Build history of the part. All positions in model axes, mm. Face numbers are marked on the shaded views. A direction names the side the tool comes from. Round coordinates to 2 decimals unless told otherwise and drop trailing zeros. Order: outer loops, then holes, each group sorted by start corner. A loop starts at its lowest first (then second) coordinate and runs counter-clockwise, first axis right, second up. Notation, with made-up numbers: M 84,53 L 104,53 A13 cw 104,62 Z; hole C -27.75,-25 d8. An arc over 180 degrees is marked long. Use CSV: the item, a comma, the result in double quotes.
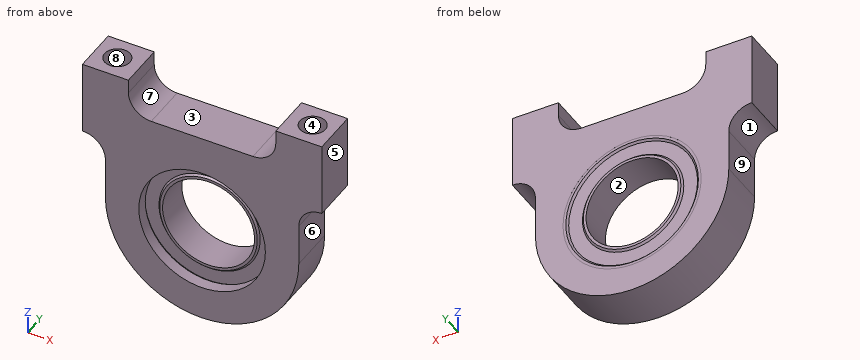
from build123d import *

# Parameters (mm, degrees)
SKETCH1_R                       = 8.73125
BOSS_EXTRUDE1_DEPTH             = 6.35
SKETCH2_R                       = 9.525
CUT_EXTRUDE1_DEPTH              = 4.7625
SKETCH3_R                       = 9.525
SKETCH3_R_2                     = 8.89
BOSS_EXTRUDE2_DEPTH             = 4.75996
CHAMFER1_SIZE                   = 0.254
SKETCH5_R                       = 6.985
SKETCH5_R_2                     = 6.35
BOSS_EXTRUDE3_DEPTH             = 4.75996
CHAMFER2_SIZE                   = 0.254
SKETCH6_R                       = 8.89
SKETCH6_R_2                     = 6.985
BOSS_EXTRUDE4_DEPTH             = 4.25196
F_6_32_TAPPED_HOLE1_D           = 2.7051
F_6_32_TAPPED_HOLE1_DEPTH       = 9.398
F_6_32_TAPPED_HOLE1_CBORE_D     = 3.5052
F_6_32_TAPPED_HOLE1_CBORE_DEPTH = 7.0104
F_6_32_TAPPED_HOLE1_TIP         = 0.81269403


with BuildPart() as part:
    # Sketch1 → Boss-Extrude1 (new body)
    with BuildSketch(Plane(origin=(0, 0, 0), x_dir=(1, 0, 0), z_dir=(0, 1, 0))):
        with BuildLine():
            Line((-13.335, 0), (-13.335, -5.7404))
            ThreePointArc((-13.335, -5.7404), (-14.257496482, -7.967503518), (-16.4846, -8.89))
            Line((-16.4846, -8.89), (-16.51, -8.89))
            Line((-16.51, -8.89), (-16.51, -19.05))
            Line((-16.51, -19.05), (-10.16, -19.05))
            Line((-10.16, -19.05), (-10.16, -17.1196))
            ThreePointArc((-10.16, -17.1196), (-9.237503518, -14.892496482), (-7.0104, -13.97))
            Line((-7.0104, -13.97), (7.0104, -13.97))
            ThreePointArc((7.0104, -13.97), (9.237503518, -14.892496482), (10.16, -17.1196))
            Line((10.16, -17.1196), (10.16, -19.05))
            Line((10.16, -19.05), (16.51, -19.05))
            Line((16.51, -19.05), (16.51, -8.89))
            Line((16.51, -8.89), (16.4846, -8.89))
            ThreePointArc((16.4846, -8.89), (14.257496482, -7.967503518), (13.335, -5.7404))
            Line((13.335, -5.7404), (13.335, 0))
            ThreePointArc((13.335, 0), (0, 13.335), (-13.335, 0))
        make_face()
        Circle(SKETCH1_R, mode=Mode.SUBTRACT)
    extrude(amount=BOSS_EXTRUDE1_DEPTH)

    # Sketch2 → Cut-Extrude1 (cut)
    with BuildSketch(Plane(origin=(0, 6.35, 0), x_dir=(1, 0, 0), z_dir=(0, 1, 0))):
        Circle(SKETCH2_R)
    extrude(amount=-CUT_EXTRUDE1_DEPTH, mode=Mode.SUBTRACT)

    # Sketch3 → Boss-Extrude2 (add)
    with BuildSketch(Plane(origin=(0, 1.5875, 0), x_dir=(-1, 0, 0), z_dir=(0, 1, 0))):
        Circle(SKETCH3_R)
        Circle(SKETCH3_R_2, mode=Mode.SUBTRACT)
    extrude(amount=BOSS_EXTRUDE2_DEPTH)

    # Chamfer1
    chamfer1_edges = [part.edges().sort_by_distance(p)[0] for p in [
        (8.89, 6.34746, 0),
    ]]
    chamfer(chamfer1_edges, length=CHAMFER1_SIZE)



with BuildPart() as body_2:
    # Sketch5 → Boss-Extrude3 (new body)
    with BuildSketch(Plane(origin=(0, 1.5875, 0), x_dir=(-1, 0, 0), z_dir=(0, 1, 0))):
        Circle(SKETCH5_R)
        Circle(SKETCH5_R_2, mode=Mode.SUBTRACT)
    extrude(amount=BOSS_EXTRUDE3_DEPTH)

    # Chamfer2
    chamfer2_edges = [body_2.edges().sort_by_distance(p)[0] for p in [
        (6.985, 1.5875, 0),
        (6.985, 6.34746, 0),
    ]]
    chamfer(chamfer2_edges, length=CHAMFER2_SIZE)


with BuildPart() as part_1:
    add(part.part)

    add(body_2.part)  # Boss-Extrude4 merges body 2
    # Sketch6 → Boss-Extrude4 (add)
    with BuildSketch(Plane(origin=(0, 6.09346, 0), x_dir=(-1, 0, 0), z_dir=(0, 1, 0))):
        Circle(SKETCH6_R)
        Circle(SKETCH6_R_2, mode=Mode.SUBTRACT)
    extrude(amount=-BOSS_EXTRUDE4_DEPTH)

    # #6-32 Tapped Hole1
    with Locations(Plane.XY.offset(19.05)):
        with Locations((-13.470384182, 3.175), (13.470384182, 3.175)):
            CounterBoreHole(F_6_32_TAPPED_HOLE1_D / 2, F_6_32_TAPPED_HOLE1_CBORE_D / 2, F_6_32_TAPPED_HOLE1_CBORE_DEPTH, depth=F_6_32_TAPPED_HOLE1_DEPTH)
            with Locations((0, 0, -(F_6_32_TAPPED_HOLE1_DEPTH + F_6_32_TAPPED_HOLE1_TIP / 2))):  # 118° drill point
                Cone(0, F_6_32_TAPPED_HOLE1_D / 2, F_6_32_TAPPED_HOLE1_TIP, mode=Mode.SUBTRACT)


solid = part_1.part
(1) Tool access for the marked faces 5, 6, 7, 8 and 9: list every direction of +Z, -Z, +X, -X, +Y, -Y with a clear straight run to the whole face (end or side of a thin tool).
Answer block:
face 5,"+Z, -Z, +X, +Y, -Y"
face 6,"-Z, +X, +Y, -Y"
face 7,"+Z, +Y, -Y"
face 8,"+Z"
face 9,"-Z, -X, +Y, -Y"
(2) Two-plate mould, pull along Z, no slides. Class the marked faces 1, 2, 3 and 4: released by +Z, released by -Z, zero draft, split by the parting line, or undercut.
Answer block:
face 1,"released by -Z"
face 2,"undercut"
face 3,"released by +Z"
face 4,"zero draft"
(3) Cut at C-C, the plane z = 14.5. Give the cut face in (x, y) (3 decimals), and give its area (3 significant figures).
Answer block:
outline,"M -16.51,0 L -8.759,0 L -8.759,6.35 L -16.51,6.35 Z; M 8.759,0 L 16.51,0 L 16.51,6.35 L 8.759,6.35 Z; hole C -13.47,3.175 d3.505; hole C 13.47,3.175 d3.505"
area,"79.1 mm²"
(4) Cut at D-D, the plane y = 5.5. Give the cut face in (x, z) (3 decimals), and give its area (3 significant figures).
Answer block:
outline,"M -16.51,8.89 L -16.485,8.89 A3.15 cw -13.335,5.74 L -13.335,0 A13.335 ccw 13.335,0 L 13.335,5.74 A3.15 cw 16.485,8.89 L 16.51,8.89 L 16.51,19.05 L 10.16,19.05 L 10.16,17.12 A3.15 cw 7.01,13.97 L -7.01,13.97 A3.15 cw -10.16,17.12 L -10.16,19.05 L -16.51,19.05 Z; hole C 0,0 d12.7"
area,"631 mm²"
(5) Drop flat-ended pins along their axis: pin 1 (7.5 mm diameter, centred on x = 0, z = 0, fed in from +Y); pin 2 (15 mm diameter, centred on x = 0.5, z = 1, fed in from -Y); pin 3 (1.8 mm diameter, centred on x = 13, y = 3, fed in from +Z); pin 4 (2 mm diameter, centred on y = 0.5, z = 6, fed in from +X). Give the stop position or say it passes through.
Answer block:
pin 1,"passes through"
pin 2,"stops at y = 1.59"
pin 3,"stops at z = 12.04"
pin 4,"stops at x = 13.6"
(6) Wall check: line 1 (X direction, y = 4.75, z = 18); line 2 (Z direction, x = 0, y = 6.3) (3 decimals); line 3 (X direction, y = 4.25, z = 10). Give the ranges that are in metal, low to high. Write a range as from..to.
Answer block:
line 1,"x = -16.51..-14.24, -12.7..-10.16, 10.16..12.7, 14.24..16.51"
line 2,"z = -13.335..-9.097, -6.778..-6.35, 6.35..6.778, 9.097..13.97"
line 3,"x = -16.51..-14.29, -12.65..12.65, 14.29..16.51"
